CAD build for the part. Positions are in the model's coordinates, mm. A direction names the side the tool comes from. Give positions to 0.01 mm unless a question says otherwise; leave off trailing zeros. Loops run counter-clockwise (first coordinate to the right, second up) from the corner with the lowest first, then second, coordinate; pieces in that order, holes last.
```python
from build123d import *

# Parameters (mm, degrees)
SKETCH1_W             = 12.7
SKETCH1_H             = 3.937
BOSS_EXTRUDE1_DEPTH   = 9.525
F_4_CLEARANCE_HOLE1_D = 2.9464
BOSS_EXTRUDE3_DEPTH   = 9.144


with BuildPart() as part:
    # Sketch1 → Boss-Extrude1 (new body)
    with BuildSketch(Plane(origin=(0, 0, 0), x_dir=(1, 0, 0), z_dir=(0, 1, 0))):
        Rectangle(SKETCH1_W, SKETCH1_H)
    extrude(amount=-BOSS_EXTRUDE1_DEPTH)

    # #4 Clearance Hole1 (through all)
    with Locations(Plane.XY.offset(1.9685)):
        with Locations((0, -3.1115)):
            Hole(F_4_CLEARANCE_HOLE1_D / 2)

    # Sketch8 → Boss-Extrude3 (add)
    with BuildSketch(Plane(origin=(-1.778, 0, 4.572), x_dir=(-1, 0, 0), z_dir=(0, 0, -1))):
        with BuildLine():
            Line((4.572, -15.875), (4.572, -9.525))
            Line((4.572, -9.525), (-8.128, -9.525))
            Line((-8.128, -9.525), (-8.128, -15.875))
            ThreePointArc((-8.128, -15.875), (-1.778, -22.225), (4.572, -15.875))
        make_face()
    extrude(amount=BOSS_EXTRUDE3_DEPTH)


solid = part.part
```
1. Saw through at C-C, the plane x = -4. List the corners of the cut face in (y, z) (1 decimal), and give its area (3 significant figures).
Responses:
outline: (-20.8, -4.6) - (-9.5, -4.6) - (-9.5, -2) - (0, -2) - (0, 2) - (-9.5, 2) - (-9.5, 4.6) - (-20.8, 4.6) - close
area: 141 mm2
2. Drop flat-ended pins along their axis: pin 1 (1.5 mm diameter, centred on x = 4, z = 1, fed in from +Y); pin 2 (5 mm diameter, centred on x = -4, z = -2, fed in from -Y); pin 3 (4 mm diameter, centred on x = 4, z = -2.5, fed in from -Y); pin 4 (3 mm diameter, centred on x = 0, z = 3.5, fed in from +Y) (3 decimals). Give the stop position or say it passes through.
Responses:
pin 1: stops at y = 0
pin 2: stops at y = -22.05
pin 3: stops at y = -21.9
pin 4: stops at y = -9.525
3. Saw through at D-D, the plane y = -5.5. List the corners of the cut face in (x, z).
Responses:
outline: (-6.35, -1.97) - (6.35, -1.97) - (6.35, 1.97) - (-6.35, 1.97) - close
4. Pull direction X, two halves, no side cores. Call faces 1 (the face through (-6.35, -10, 0)), 2 (the face through (0, -9.525, -3)), 3 (the face through (0.32, -4.55, -0.03)): released by +X, released by -X, zero draft, split by the parting line, or undercut.
Responses:
face 1: released by -X
face 2: zero draft
face 3: undercut
5. Probe line 1 along Y through (x, z) = (0, -1.1) (3 decimals); line 2 along Z through (x, y) = (-0.5, -0.75); line 3 along Y through (x, z) = (-0.5, -1). List the from-to ranges inside material, lowest first.
Responses:
line 1: y = -22.225 to -4.585, -1.638 to 0
line 2: z = -1.97 to 1.97
line 3: y = -22.21 to -4.5, -1.73 to 0
6. Tool access for faces 4 (the face through (0, 0, 0)), 5 (the face through (0, -5, 1.968)), 6 (the face through (0, -5, -1.968)): list every direction of +Z, -Z, +X, -X, +Y, -Y with a clear straight run to the whole face (end or side of a thin tool).
Responses:
face 4: +Z, -Z, +X, -X, +Y
face 5: +Z, +X, -X, +Y
face 6: -Z, +X, -X, +Y
7. Saw through at A-A, the plane x = 0. List the corners of the cut face in (y, z) (1 decimal).
Responses:
outline: (-22.2, -4.6) - (-9.5, -4.6) - (-9.5, -2) - (-4.6, -2) - (-4.6, 2) - (-9.5, 2) - (-9.5, 4.6) - (-22.2, 4.6) - close; (-1.6, -2) - (0, -2) - (0, 2) - (-1.6, 2) - close
